Part model, mm, in its own coordinate system. A direction names the side the tool comes from. Give positions to 0.01 mm unless a question says otherwise; leave off trailing zeros. Write each loop counter-clockwise with the first axis right and the second up, starting at its lowest first coordinate (ties: lowest second). Pieces come first, ordered by that corner, then holes.
```python
from build123d import *

# Parameters (mm, degrees)
F0_W     = 12.5
F0_H     = 16
F0_R     = 1.25
F1_DEPTH = 1.5
F2_W     = 1.5
F2_H     = 16
F3_DEPTH = 5.5
F5_DEPTH = 3
F4_W     = 1.5
F4_H     = 16
F6_DEPTH = 1.5
F8_DEPTH = 4


# Not quite as in the source:
# - a feature of the source that left no trace in its solid (it failed there, or was rolled back) is left out


with BuildPart() as f1:
    # F0 (on Top) → F1 (new body)
    with BuildSketch(Plane.XY):
        with Locations((-6.25, -8)):
            Rectangle(F0_W, F0_H)
        with Locations((-3.25, -13)):
            Circle(F0_R, mode=Mode.SUBTRACT)
        with Locations((-3.25, -3)):
            Circle(F0_R, mode=Mode.SUBTRACT)
    extrude(amount=F1_DEPTH)

    # F2 (on face) → F3 (join)
    with BuildSketch(Plane(origin=(0, 0, 0), x_dir=(1, 0, 0), z_dir=(0, 0, -1))):
        with Locations((-11.75, 8)):
            Rectangle(F2_W, F2_H)
    extrude(amount=F3_DEPTH)

    # F4 (on face) → F5 (join)
    with BuildSketch(Plane(origin=(0, 0, -5.5), x_dir=(1, 0, 0), z_dir=(0, 0, -1))):
        Polygon((-11, 16), (-11, 19.875), (-29.75, 19.875), (-29.75, -3.875), (-11, -3.875), (-11, 0), (-12.5, 0), (-12.5, -2.375), (-28.25, -2.375), (-28.25, 18.375), (-12.5, 18.375), (-12.5, 16), align=None)
    extrude(amount=-F5_DEPTH)

    # F4 (on face) → F6 (join)
    with BuildSketch(Plane(origin=(0, 0, -5.5), x_dir=(1, 0, 0), z_dir=(0, 0, -1))):
        Polygon((-11, 16), (-11, 19.875), (-29.75, 19.875), (-29.75, -3.875), (-11, -3.875), (-11, 0), (-12.5, 0), (-12.5, -2.375), (-28.25, -2.375), (-28.25, 18.375), (-12.5, 18.375), (-12.5, 16), align=None)
        with Locations((-11.75, 8)):
            Rectangle(F4_W, F4_H)
        Polygon((-12.5, 0), (-12.5, 16), (-12.5, 18.375), (-28.25, 18.375), (-28.25, -2.375), (-12.5, -2.375), align=None)
        with BuildLine():
            Line((-13.375, 11.125), (-13.375, 4.875))
            ThreePointArc((-13.375, 4.875), (-15, 3.25), (-16.625, 4.875))
            Line((-16.625, 4.875), (-16.625, 11.125))
            ThreePointArc((-16.625, 11.125), (-15, 12.75), (-13.375, 11.125))
        make_face(mode=Mode.SUBTRACT)
    extrude(amount=F6_DEPTH)

    # F7 (on face) → F8 (join)
    with BuildSketch(Plane.YZ.offset(-11)):
        Polygon((0, 0), (-16, 0), (-16, -2.5), (-16, -7), (0, -7), (0, -2.5), align=None)
    extrude(amount=F8_DEPTH)


solid = f1.part
```
1) Saw through at A-A, the plane x = -3.25. Write the cut outline in (y, z).
Answers follow:
outline: (-16, 0) - (-14.25, 0) - (-14.25, 1.5) - (-16, 1.5) - close; (-11.75, 0) - (-4.25, 0) - (-4.25, 1.5) - (-11.75, 1.5) - close; (-1.75, 0) - (0, 0) - (0, 1.5) - (-1.75, 1.5) - close
2) Two-plate mould, pull along Y, no slides. Class faces 1 (the face through (-21, 3.875, -5)), 2 (the face through (-16.625, -8, -6)), 3 (the face through (-19, -8, -7)): +Y half, -Y half, draft (parallel to the pull), parting line (faces both ways), or undercut.
Answers follow:
face 1: +Y half
face 2: undercut
face 3: draft
3) Saw through at B-B, the plane z = -3. Write the cut outline in (x, y) (3 decimals).
Answers follow:
outline: (-29.75, -19.875) - (-11, -19.875) - (-11, -16) - (-7, -16) - (-7, 0) - (-11, 0) - (-11, 3.875) - (-29.75, 3.875) - close; hole (-28.25, -18.375) - (-12.5, -18.375) - (-12.5, 2.375) - (-28.25, 2.375) - close
4) 3-axis set-ups, long thin cutter, end or side, ignore diameter. For faces 4 (the face through (-28.25, -8, -4)), 5 (the face through (-11, -18, -5)), 6 (the face through (-14.96, -3.25, -6.24)), 7 (the face through (-4, -8, 0)): which of +Z, -Z, +X, -X, +Y, -Y reach the whole face in a straight line?
Answers follow:
face 4: +Z
face 5: +Z, -Z, +X, -Y
face 6: +Z, -Z
face 7: -Z, +X, +Y, -Y
5) Saw through at C-C, the plane x = -15. Write the cut outline in (y, z) (3 decimals).
Answers follow:
outline: (-19.875, -7) - (-12.75, -7) - (-12.75, -5.5) - (-18.375, -5.5) - (-18.375, -2.5) - (-19.875, -2.5) - close; (-3.25, -7) - (3.875, -7) - (3.875, -2.5) - (2.375, -2.5) - (2.375, -5.5) - (-3.25, -5.5) - close
6) Saw through at D-D, the plane y = -9.5. Write the cut outline in (x, z) (3 decimals).
Answers follow:
outline: (-29.75, -7) - (-16.625, -7) - (-16.625, -5.5) - (-28.25, -5.5) - (-28.25, -2.5) - (-29.75, -2.5) - close; (-13.375, -7) - (-7, -7) - (-7, 0) - (0, 0) - (0, 1.5) - (-12.5, 1.5) - (-12.5, -5.5) - (-13.375, -5.5) - close
7) Wall check: L1, parallel to Y at x = -3.25, z = 0.9; L2, parallel to Y at x = -17.5, z = -4.75 (3 decimals); L3, parallel to X at y = -15.75, z = -3. Give the ranges that are in metal, low to high.
Answers follow:
L1: y = -16 to -14.25, -11.75 to -4.25, -1.75 to 0
L2: y = -19.875 to -18.375, 2.375 to 3.875
L3: x = -29.75 to -28.25, -12.5 to -7
8) Pin check, flat tips, straight feed: pin 1 Ø4 at (x, z) = (-5, -1.5) entering from +Y; pin 2 Ø1.9 at (y, z) = (-18, -5.5) entering from +X; pin 3 Ø1.5 at (y, z) = (-11.5, -3.5) entering from +X. Stop position of each tip, or through.
Answers follow:
pin 1: stops at y = 0
pin 2: stops at x = -11
pin 3: stops at x = -7
